```python
from build123d import *

# Parameters (mm, degrees)
SKETCH_2_W          = 30.48
SKETCH_2_H          = 30.48
EXTRUDE_1_DEPTH     = 8.6
SKETCH_3_R          = 3.1
CUT_EXTRUDE_1_DEPTH = 30.48
SKETCH_4_R          = 3.1
CUT_EXTRUDE_2_DEPTH = 30.48
SKETCH_5_R          = 1.6
CUT_EXTRUDE_3_DEPTH = 9.6
FILLET_2_R          = 2.54


with BuildPart() as part:
    # 草图2 → 凸台-拉伸1 (new body)
    with BuildSketch(Plane(origin=(0, 0, 0), x_dir=(1, 0, 0), z_dir=(0, 1, 0))):
        Rectangle(SKETCH_2_W, SKETCH_2_H)
    extrude(amount=EXTRUDE_1_DEPTH)

    # 草图3 → 切除-拉伸1 (cut)
    with BuildSketch(Plane.XY.offset(15.24)):
        with Locations((0, 8.7)):
            Circle(SKETCH_3_R)
    extrude(amount=-CUT_EXTRUDE_1_DEPTH, mode=Mode.SUBTRACT)

    # 草图4 → 切除-拉伸2 (cut)
    with BuildSketch(Plane(origin=(15.24, 0, 0), x_dir=(0, 0, -1), z_dir=(1, 0, 0))):
        with Locations((0, -0.1)):
            Circle(SKETCH_4_R)
    extrude(amount=-CUT_EXTRUDE_2_DEPTH, mode=Mode.SUBTRACT)

    # 草图5 → 切除-拉伸3 (cut, through all)
    with BuildSketch(Plane.XZ):
        with Locations((-11.24, 11.24)):
            Circle(SKETCH_5_R)
        with Locations((11.24, 11.24)):
            Circle(SKETCH_5_R)
        with Locations((11.24, -11.24)):
            Circle(SKETCH_5_R)
        with Locations((-11.24, -11.24)):
            Circle(SKETCH_5_R)
    extrude(amount=-CUT_EXTRUDE_3_DEPTH, mode=Mode.SUBTRACT)

    # 圆角2
    fillet_2_edges = [part.edges().sort_by_distance(p)[0] for p in [
        (15.24, 4.3, 15.24),
        (-15.24, 4.3, 15.24),
        (-15.24, 4.3, -15.24),
        (15.24, 4.3, -15.24),
    ]]
    fillet(fillet_2_edges, radius=FILLET_2_R)


solid = part.part
```
Read the model definition and answer for the solid it produces. Units are mm, in the model's axes. Round coordinates to 2 decimals unless told otherwise and drop trailing zeros. Write each loop counter-clockwise with the first axis right and the second up, starting at its lowest first coordinate (ties: lowest second). Pieces come first, ordered by that corner, then holes. Notation, with made-up numbers: (-5, -28) -> (9, -28) arc R17 ccw to (9, -9) -> close; hole circle Ø11 at (33, 85.5). An arc over 180 degrees is marked (long way). Answer in a Markdown table with one row per item. Add a question column.
1) Consider line 1 (Z direction, x = -11.24, y = 6.5); line 2 (X direction, y = 4.5, z = 11.5); line 3 (X direction, y = 4.75, z = -12.5). Determine where each line is inside the solid, lowest interval first.
2) Find section A-A, the plane y = 1.5. Determine the outline of the cut face in (x, z), and give its area (3 significant figures).
3) Find section D-D, the plane y = 5. Determine the outline of the cut face in (x, z), and give its area (3 significant figures).
4) Find section C-C, the plane z = -10.5. Determine the outline of the cut face in (x, y), and give its area (3 significant figures).
5) Find section B-B, the plane x = -11.24. Determine the outline of the cut face in (y, z).
6) Determine the mould class of faces 1 (the face through (-11.448, 4.24, 12.826)), 2 (the face through (14.476, 4.36, 14.516)), 3 (the face through (-9, 8.6, 0)) for opening direction Z: pulls with the +Z half, pulls with the -Z half, needs draft (parallel to the pull), parting line crosses it, or undercut.
Findings below:
| question | item | result |
|---|---|---|
| 1 | line 1 | -15.24 to -12.84, -9.64 to 9.64, 12.84 to 15.24 |
| 1 | line 2 | -15.24 to -12.82, -9.66 to 9.66, 12.82 to 15.24 |
| 1 | line 3 | -15.24 to -12.23, -10.25 to 10.25, 12.23 to 15.24 |
| 2 | outline | (-15.24, -12.7) arc R2.54 ccw to (-12.7, -15.24) -> (12.7, -15.24) arc R2.54 ccw to (15.24, -12.7) -> (15.24, -2.66) -> (-15.24, -2.66) -> close; (-15.24, 2.66) -> (15.24, 2.66) -> (15.24, 12.7) arc R2.54 ccw to (12.7, 15.24) -> (-12.7, 15.24) arc R2.54 ccw to (-15.24, 12.7) -> close; hole circle Ø3.2 at (-11.24, -11.24); hole circle Ø3.2 at (-11.24, 11.24); hole circle Ø3.2 at (11.24, -11.24); hole circle Ø3.2 at (11.24, 11.24) |
| 2 | area | 729 mm² |
| 3 | outline | (-15.24, -12.7) arc R2.54 ccw to (-12.7, -15.24) -> (12.7, -15.24) arc R2.54 ccw to (15.24, -12.7) -> (15.24, 12.7) arc R2.54 ccw to (12.7, 15.24) -> (-12.7, 15.24) arc R2.54 ccw to (-15.24, 12.7) -> close; hole circle Ø3.2 at (-11.24, -11.24); hole circle Ø3.2 at (-11.24, 11.24); hole circle Ø3.2 at (11.24, -11.24); hole circle Ø3.2 at (11.24, 11.24) |
| 3 | area | 891 mm² |
| 4 | outline | (-15.24, 0) -> (-12.66, 0) -> (-12.66, 8.6) -> (-15.24, 8.6) -> close; (-9.82, 0) -> (9.82, 0) -> (9.82, 8.6) -> (3.1, 8.6) arc R3.1 cw to (-3.1, 8.6) -> (-9.82, 8.6) -> close; (12.66, 0) -> (15.24, 0) -> (15.24, 8.6) -> (12.66, 8.6) -> close |
| 4 | area | 199 mm² |
| 5 | outline | (0, -15.24) -> (8.6, -15.24) -> (8.6, -12.84) -> (0, -12.84) -> close; (0, -9.64) -> (8.6, -9.64) -> (8.6, 9.64) -> (0, 9.64) -> (0, 3.1) arc R3.1 cw to (0, -3.1) -> close; (0, 12.84) -> (8.6, 12.84) -> (8.6, 15.24) -> (0, 15.24) -> close |
| 6 | face 1 | undercut |
| 6 | face 2 | pulls with the +Z half |
| 6 | face 3 | needs draft |
